from build123d import *

# Parameters (mm, degrees)
F0_R     = 2.1
F0_R_2   = 9.25
F1_DEPTH = 1.2
F2_R     = 0.3


with BuildPart() as f1:
    # F0 (on Top) → F1 (new body)
    with BuildSketch(Plane.XY):
        with BuildLine():
            ThreePointArc((-77.110974, 15.5), (-78.516861, 18.894113), (-81.910974, 20.3))
            ThreePointArc((-81.910974, 20.3), (-85.861289, 18.226722), (-86.399062, 13.797923))
            ThreePointArc((-86.399062, 13.797923), (-81.045764, 10.778622), (-77.110974, 15.5))
        make_face()
        with Locations((-81.910974, 15.5)):
            Circle(F0_R, mode=Mode.SUBTRACT)
        with BuildLine():
            ThreePointArc((-78.436359, -7.198369), (-76.162026, 11.531763), (-59.455487, 20.3))
            Line((-59.455487, 20.3), (-81.910974, 20.3))
            ThreePointArc((-81.910974, 20.3), (-78.516861, 18.894113), (-77.110974, 15.5))
            ThreePointArc((-77.110974, 15.5), (-81.045764, 10.778622), (-86.399062, 13.797923))
            Line((-86.399062, 13.797923), (-78.436359, -7.198369))
        make_face()
        with BuildLine():
            ThreePointArc((-59.455487, -19), (-46.020458, -13.435029), (-40.455487, 0))
            ThreePointArc((-40.455487, 0), (-46.020458, 13.435029), (-59.455487, 19))
            ThreePointArc((-59.455487, 19), (-78.455487, 0), (-59.455487, -19))
        make_face()
        with BuildLine():
            ThreePointArc((-58.74838, -17.74838), (-59.455487, -18.041273), (-60.162594, -17.74838))
            Line((-60.162594, -17.74838), (-67.09224, -10.818734))
            ThreePointArc((-67.09224, -10.818734), (-67.385133, -10.111627), (-67.09224, -9.40452))
            Line((-67.09224, -9.40452), (-60.162594, -2.474874))
            ThreePointArc((-60.162594, -2.474874), (-59.455487, -2.181981), (-58.74838, -2.474874))
            Line((-58.74838, -2.474874), (-51.818734, -9.40452))
            ThreePointArc((-51.818734, -9.40452), (-51.525841, -10.111627), (-51.818734, -10.818734))
            Line((-51.818734, -10.818734), (-58.74838, -17.74838))
        make_face(mode=Mode.SUBTRACT)
        with BuildLine():
            ThreePointArc((-70.274221, 7.636753), (-69.567114, 7.929646), (-68.860007, 7.636753))
            Line((-68.860007, 7.636753), (-61.930361, 0.707107))
            ThreePointArc((-61.930361, 0.707107), (-61.637468, 0), (-61.930361, -0.707107))
            Line((-61.930361, -0.707107), (-68.860007, -7.636753))
            ThreePointArc((-68.860007, -7.636753), (-69.567114, -7.929646), (-70.274221, -7.636753))
            Line((-70.274221, -7.636753), (-77.203867, -0.707107))
            ThreePointArc((-77.203867, -0.707107), (-77.49676, 0), (-77.203867, 0.707107))
            Line((-77.203867, 0.707107), (-70.274221, 7.636753))
        make_face(mode=Mode.SUBTRACT)
        with BuildLine():
            Line((-48.636753, 7.636753), (-41.707107, 0.707107))
            ThreePointArc((-41.707107, 0.707107), (-41.414214, 0), (-41.707107, -0.707107))
            Line((-41.707107, -0.707107), (-48.636753, -7.636753))
            ThreePointArc((-48.636753, -7.636753), (-49.34386, -7.929646), (-50.050967, -7.636753))
            Line((-50.050967, -7.636753), (-56.980613, -0.707107))
            ThreePointArc((-56.980613, -0.707107), (-57.273506, 0), (-56.980613, 0.707107))
            Line((-56.980613, 0.707107), (-50.050967, 7.636753))
            ThreePointArc((-50.050967, 7.636753), (-49.34386, 7.929646), (-48.636753, 7.636753))
        make_face(mode=Mode.SUBTRACT)
        with BuildLine():
            ThreePointArc((-51.818734, 10.818734), (-51.525841, 10.111627), (-51.818734, 9.40452))
            Line((-51.818734, 9.40452), (-58.74838, 2.474874))
            ThreePointArc((-58.74838, 2.474874), (-59.455487, 2.181981), (-60.162594, 2.474874))
            Line((-60.162594, 2.474874), (-67.09224, 9.40452))
            ThreePointArc((-67.09224, 9.40452), (-67.385133, 10.111627), (-67.09224, 10.818734))
            Line((-67.09224, 10.818734), (-60.162594, 17.74838))
            ThreePointArc((-60.162594, 17.74838), (-59.455487, 18.041273), (-58.74838, 17.74838))
            Line((-58.74838, 17.74838), (-51.818734, 10.818734))
        make_face(mode=Mode.SUBTRACT)
        with BuildLine():
            Line((-40.284814, 19), (-52.30776, 19))
            ThreePointArc((-52.30776, 19), (-42.764339, 11.554028), (-39.155487, 0))
            ThreePointArc((-39.155487, 0), (-42.764339, -11.554028), (-52.30776, -19))
            Line((-52.30776, -19), (-40.284814, -19))
            ThreePointArc((-40.284814, -19), (-40.394113, -12.105887), (-33.5, -12.215186))
            Line((-33.5, -12.215186), (-33.5, 0))
            Line((-33.5, 0), (-33.5, 12.215186))
            ThreePointArc((-33.5, 12.215186), (-40.394113, 12.105887), (-40.284814, 19))
        make_face()
        with BuildLine():
            ThreePointArc((-59.455487, 19), (-46.020458, 13.435029), (-40.455487, 0))
            ThreePointArc((-40.455487, 0), (-46.020458, -13.435029), (-59.455487, -19))
            Line((-59.455487, -19), (-52.30776, -19))
            ThreePointArc((-52.30776, -19), (-42.764339, -11.554028), (-39.155487, 0))
            ThreePointArc((-39.155487, 0), (-42.764339, 11.554028), (-52.30776, 19))
            Line((-52.30776, 19), (-59.455487, 19))
        make_face()
        with BuildLine():
            ThreePointArc((-59.455487, -19), (-78.455487, 0), (-59.455487, 19))
            Line((-59.455487, 19), (-52.30776, 19))
            ThreePointArc((-52.30776, 19), (-55.822995, 19.972356), (-59.455487, 20.3))
            ThreePointArc((-59.455487, 20.3), (-76.162026, 11.531763), (-78.436359, -7.198369))
            ThreePointArc((-78.436359, -7.198369), (-74.258704, -13.890816), (-67.845188, -18.485208))
            ThreePointArc((-67.845188, -18.485208), (-63.747356, -19.841115), (-59.455487, -20.3))
            ThreePointArc((-59.455487, -20.3), (-55.822995, -19.972356), (-52.30776, -19))
            Line((-52.30776, -19), (-59.455487, -19))
        make_face()
        with BuildLine():
            ThreePointArc((-59.455487, 20.3), (-55.822995, 19.972356), (-52.30776, 19))
            Line((-52.30776, 19), (-40.284814, 19))
            ThreePointArc((-40.284814, 19), (-38.766352, 19.963183), (-37, 20.3))
            Line((-37, 20.3), (-59.455487, 20.3))
        make_face()
        with BuildLine():
            ThreePointArc((-37, 20.3), (-38.766352, 19.963183), (-40.284814, 19))
            ThreePointArc((-40.284814, 19), (-40.394113, 12.105887), (-33.5, 12.215186))
            ThreePointArc((-33.5, 12.215186), (-32.536817, 13.733648), (-32.2, 15.5))
            ThreePointArc((-32.2, 15.5), (-33.605887, 18.894113), (-37, 20.3))
        make_face()
        with Locations((-37, 15.5)):
            Circle(F0_R, mode=Mode.SUBTRACT)
        with BuildLine():
            ThreePointArc((-32.2, 15.5), (-32.536817, 13.733648), (-33.5, 12.215186))
            Line((-33.5, 12.215186), (-33.5, 0))
            Line((-33.5, 0), (-32.2, 0))
            Line((-32.2, 0), (-32.2, 4.854651))
            Line((-32.2, 4.854651), (-32.2, 15.5))
        make_face()
        with BuildLine():
            ThreePointArc((-33.5, -12.215186), (-40.394113, -12.105887), (-40.284814, -19))
            ThreePointArc((-40.284814, -19), (-38.766352, -19.963183), (-37, -20.3))
            ThreePointArc((-37, -20.3), (-33.605887, -18.894113), (-32.2, -15.5))
            ThreePointArc((-32.2, -15.5), (-32.536817, -13.733648), (-33.5, -12.215186))
        make_face()
        with Locations((-37, -15.5)):
            Circle(F0_R, mode=Mode.SUBTRACT)
        with BuildLine():
            Line((-40.284814, -19), (-52.30776, -19))
            ThreePointArc((-52.30776, -19), (-55.822995, -19.972356), (-59.455487, -20.3))
            Line((-59.455487, -20.3), (-37, -20.3))
            ThreePointArc((-37, -20.3), (-38.766352, -19.963183), (-40.284814, -19))
        make_face()
        with BuildLine():
            Line((-37, -20.3), (-59.455487, -20.3))
            ThreePointArc((-59.455487, -20.3), (-63.747356, -19.841115), (-67.845188, -18.485208))
            Line((-67.845188, -18.485208), (-24.199465, -38.294266))
            ThreePointArc((-24.199465, -38.294266), (-30.415777, -25.13497), (-18.44759, -16.854144))
            Line((-18.44759, -16.854144), (-29.493976, -15.766451))
            ThreePointArc((-29.493976, -15.766451), (-31.422828, -14.795594), (-32.2, -12.78089))
            Line((-32.2, -12.78089), (-32.2, 0))
            Line((-32.2, 0), (-33.5, 0))
            Line((-33.5, 0), (-33.5, -12.215186))
            ThreePointArc((-33.5, -12.215186), (-32.536817, -13.733648), (-32.2, -15.5))
            ThreePointArc((-32.2, -15.5), (-33.605887, -18.894113), (-37, -20.3))
        make_face()
        with BuildLine():
            ThreePointArc((-18.44759, -16.854144), (-30.415777, -25.13497), (-24.199465, -38.294266))
            ThreePointArc((-24.199465, -38.294266), (-13.456724, -37.506981), (-8.3, -28.05))
            ThreePointArc((-8.3, -28.05), (-11.214395, -20.494857), (-18.44759, -16.854144))
        make_face()
        with Locations((-19.55, -28.05)):
            Circle(F0_R_2, mode=Mode.SUBTRACT)
    extrude(amount=-F1_DEPTH)

    # F2
    f2_edges = [f1.edges().sort_by_distance(p)[0] for p in [
        (-46.022326, -28.389737, -1.2),
        (-74.258704, -13.890816, -1.2),
        (-82.41771, 3.299777, -1.2),
        (-85.861289, 18.226722, -1.2),
        (-59.455487, 20.3, -1.2),
        (-33.605887, 18.894113, -1.2),
        (-32.2, 1.359555, -1.2),
        (-31.422828, -14.795594, -1.2),
        (-23.970783, -16.310298, -1.2),
        (-8.684223, -30.96503, -1.2),
    ]]
    fillet(f2_edges, radius=F2_R)


solid = f1.part
Work out the finished part from the listing and answer in its coordinate system (mm). A direction names the side the tool comes from. Coordinates: 2 decimals unless noted, no trailing zeros.
1. The part is cut by section A-A, the plane z = -0.6. State how many separate pieces and enclosed holes the cut face has, and give its area (3 significant figures).
Results list:
separate pieces: 1
enclosed holes: 8
area: 1,770 mm2
2. A flat-ended cylindrical pin translates along its axis: pin 1 (2.5 mm diameter, centred on x = -37, y = 15.5, fed in from -Z). Find the tip coordinate at first contact, or state that the pin passes through.
Results list:
pin 1: passes through
3. Consider line 1 along Y through (x, z) = (-37, -0.2); line 2 along Y through (x, z) = (-63, -1.05); line 3 along X through (y, z) = (4, -0.45). Determine where each line is inside the solid, lowest interval first.
Results list:
line 1: y = -32.48 to -17.6, -13.4 to 13.4, 17.6 to 20.3
line 2: y = -20.64 to -14.91, -5.31 to -1.78, 1.78 to 5.31, 14.91 to 20.26
line 3: x = -82.68 to -73.91, -65.22 to -61.69, -57.22 to -53.69, -45 to -32.2
4. For faces 1 (the flat face through (-51, -9, -1.2)), 2 (the flat face through (-55.235, 5.988, -0.592)), determine the directions among +Z, -Z, +X, -X, +Y, -Y from which every point of the face is accessible in a straight line to the end or side of a thin tool.
Results list:
face 1: -Z, +X, -X, +Y, -Y
face 2: +Z, -Z
5. For a pull along X with two mould halves and no side action, classify faces 3 (the flat face through (-55, 14, -1)), 4 (the flat face through (-53, -5, 0)), 5 (the flat face through (-82.473, 3.447, -0.444)) as +X half, -X half, draft (parallel to the pull), parting line (faces both ways), or undercut.
Results list:
face 3: undercut
face 4: draft
face 5: -X half
